Source: CAD feature listing. Evaluate the final solid. Frame: model axes, mm. A direction names the side the tool comes from. Coordinates: 2 decimals unless noted, no trailing zeros. Loops run counter-clockwise (first coordinate to the right, second up) from the corner with the lowest first, then second, coordinate; pieces in that order, holes last. Notation, with made-up numbers: M -28.75,67 L 26.25,67 A17 cw 26.25,95 Z; hole C 83,9 d2. An arc over 180 degrees is marked long. One line per question, with ' | ' between items. Start each with the question number.
1. Section query A-A, the plane z = 0.25. Output: boundary loops of the cut face in (x, y), and give its area (3 significant figures).
2. Section query B-B, the plane x = -1. Output: boundary loops of the cut face in (y, z), and give its area (3 significant figures).
3. Access query for faces 4 (the flat face through (0.5, 2, 0.5)), 5 (the flat face through (0, 2, 0)), 6 (the flat face through (2, -1, 0.7)). Directions: +Z, -Z, +X, -X, +Y, -Y. A direction counts if a zero-diameter tool reaches every point of the face in a straight line with its end or side. Return the directions, or none.
4. Ray query, probe 1 along Y at (x, z) = (-1, 0.5); probe 2 along X at (y, z) = (0.25, 0.7); probe 3 along Y at (x, z) = (-5.5, 0.3). Return the intervals inside material, ascending.
5. Section query C-C, the plane y = 0.25. Output: boundary loops of the cut face in (x, z), and give its area (3 significant figures).
6. Section query D-D, the plane x = -5. Output: boundary loops of the cut face in (y, z).
7. Mould query, pull axis Y, two halves, no side actions, for faces 1 (the cylindrical face through (-0.07, -1.05, 0.35)), 2 (the cylindrical face through (-1.065, 5.496, 0.493)), 3 (the flat face through (-0.5, 2.1, 0.5)). Classes: pulls with the +Y half, pulls with the -Y half, needs draft (parallel to the pull), parting line crosses it, or undercut.
8. Pin query (flat end, axial travel): P1, Ø1.5, axis at x = 3.5, y = 2, coming from the -Z side; P2, Ø0.8, axis at x = -0.5, y = 3.5, coming from the +Z side; P3, Ø0.8, axis at x = -4, y = 5, coming from the +Z side; P4, Ø0.5, axis at y = 1.5, z = 0.5, coming from the -X side. Return the tip coordinate at first contact, or that it passes through.
```python
from build123d import *

# Parameters (mm, degrees)
F0_R     = 0.25
F1_DEPTH = 0.5
F0_R_2   = 0.5
F2_DEPTH = 1
F3_DEPTH = 0.7
F4_DEPTH = 0.7
F5_DEPTH = 1.2


with BuildPart() as f1:
    # F0 (on Top) → F1 (new body)
    with BuildSketch(Plane.XY):
        with BuildLine():
            Line((-5.5, 4.5), (-1.866025, 4.5))
            ThreePointArc((-1.866025, 4.5), (-2, 5), (-1.866025, 5.5))
            Line((-1.866025, 5.5), (-5.5, 5.5))
            ThreePointArc((-5.5, 5.5), (-6, 5), (-5.5, 4.5))
        make_face()
        with Locations((-5.5, 5)):
            Circle(F0_R, mode=Mode.SUBTRACT)
    extrude(amount=F1_DEPTH)

    # F0 (on Top) → F2 (join)
    with BuildSketch(Plane.XY):
        with BuildLine():
            ThreePointArc((-1.866025, 4.5), (-1.258819, 4.034074), (-0.5, 4.133975))
            Line((-0.5, 4.133975), (-0.5, 0))
            Line((-0.5, 0), (0.5, 0))
            Line((0.5, 0), (0.5, 4.085786))
            ThreePointArc((0.5, 4.085786), (0.42388, 4.46847), (0.207107, 4.792893))
            Line((0.207107, 4.792893), (0, 5))
            ThreePointArc((0, 5), (-0.741181, 5.965926), (-1.866025, 5.5))
            ThreePointArc((-1.866025, 5.5), (-2, 5), (-1.866025, 4.5))
        make_face()
        with Locations((-1, 5)):
            Circle(F0_R_2, mode=Mode.SUBTRACT)
    extrude(amount=F2_DEPTH)

    # F0 (on Top) → F3 (join)
    with BuildSketch(Plane.XY):
        with BuildLine():
            Line((0.5, 0), (-0.5, 0))
            ThreePointArc((-0.5, 0), (-0.06066, -1.06066), (1, -1.5))
            Line((1, -1.5), (4, -1.071429))
            Line((4, -1.071429), (4, -0.071429))
            Line((4, -0.071429), (1, -0.5))
            ThreePointArc((1, -0.5), (0.646447, -0.353553), (0.5, 0))
        make_face()
    extrude(amount=F3_DEPTH)

    # F0 (on Top) → F4 (join, through all)
    with BuildSketch(Plane.XY):
        Polygon((4, -0.071429), (4, -1.071429), (4.5, -1), (4.5, 0), align=None)
    extrude(amount=F4_DEPTH)

    # F0 (on Top) → F5 (join)
    with BuildSketch(Plane.XY):
        with Locations((-5.5, 5)):
            Circle(F0_R)
    extrude(amount=F5_DEPTH)


solid = f1.part
```
Taken from the geometry:
1) outline: M -5.5,4.5 L -1.87,4.5 A1 ccw -0.5,4.13 L -0.5,0 A1.5 ccw 1,-1.5 L 4,-1.07 L 4.5,-1 L 4.5,0 L 4,-0.07 L 1,-0.5 A0.5 cw 0.5,0 L 0.5,4.09 A1 ccw 0.21,4.79 L 0,5 A1 ccw -1.87,5.5 L -5.5,5.5 A0.5 ccw Z; hole C -1,5 d1 | area: 15.9 mm^2
2) outline: M 4,0 L 4.5,0 L 4.5,1 L 4,1 Z; M 5.5,0 L 6,0 L 6,1 L 5.5,1 Z | area: 1.00 mm^2
3) face 4: +Z, -Z, +X, +Y | face 5: -Z, +X, -X, +Y, -Y | face 6: +Z, +X, -X, -Y
4) probe 1: 4 to 4.5, 5.5 to 6 | probe 2: -0.5 to 0.5 | probe 3: 4.5 to 5.5
5) outline: M -0.5,0 L 0.5,0 L 0.5,1 L -0.5,1 Z | area: 1.00 mm^2
6) outline: M 4.5,0 L 5.5,0 L 5.5,0.5 L 4.5,0.5 Z
7) face 1: pulls with the -Y half | face 2: undercut | face 3: needs draft
8) P1: through | P2: z = 1 | P3: z = 0.5 | P4: x = -0.5
